Here's how the part is built. I have some questions about the finished solid (model axes, mm). Round coordinates to 2 decimals unless told otherwise and drop trailing zeros. Write each loop counter-clockwise with the first axis right and the second up, starting at its lowest first coordinate (ties: lowest second). Pieces come first, ordered by that corner, then holes. Notation, with made-up numbers: (-22, -40) - (-3, -40) arc R23 cw to (-3, -18) - close; hole circle Ø9 at (25.5, 83.25). An arc over 180 degrees is marked (long way). One line per question, with ' | ' between items. Start each with the question number.
(1) Imagine slicing it at C-C (z = 0.8). Write out the boundary of the cut face in (x, y).
(2) Imagine slicing it at A-A (y = -6.75). Write out the boundary of the cut face in (x, z).
(3) If I drill on L1, parallel to X at y = -5, z = 0.5; L2, parallel to Y at x = 0.1, z = 0.95; L3, parallel to Z at x = -1.6, y = -3, over which ranges is the centre line in solid material (lowest first)?
(4) Imagine slicing it at D-D (x = -0.15). Write out the boundary of the cut face in (y, z).
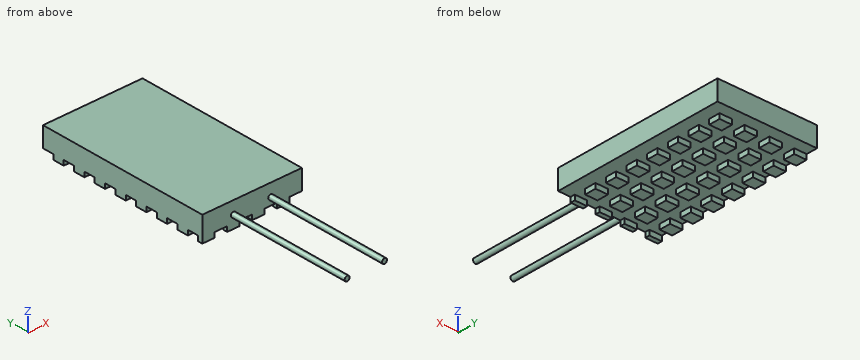
from build123d import *

# Parameters (mm, degrees)
SKETCH_1_W          = 4
SKETCH_1_H          = 7
EXTRUDE_1_DEPTH     = 1
SKETCH_2_W          = 0.5
SKETCH_2_H          = 7
CUT_EXTRUDE_2_DEPTH = 0.2
SKETCH_3_W          = 4
SKETCH_3_H          = 0.454516336
SKETCH_3_H_2        = 0.454516335
CUT_EXTRUDE_4_DEPTH = 0.2
SWEEP_1_PROFILE_R   = 0.1
SWEEP_2_PROFILE_R   = 0.1


with BuildPart() as part:
    # 草图1 → 凸台-拉伸1 (new body)
    with BuildSketch(Plane.XY):
        Rectangle(SKETCH_1_W, SKETCH_1_H)
    extrude(amount=EXTRUDE_1_DEPTH)

    # 草图2 → 切除-拉伸2 (cut)
    with BuildSketch(Plane.XY):
        with Locations((1.75, 0)):
            Rectangle(SKETCH_2_W, SKETCH_2_H)
        with Locations((0.75, 0)):
            Rectangle(SKETCH_2_W, SKETCH_2_H)
        with Locations((-0.25, 0)):
            Rectangle(SKETCH_2_W, SKETCH_2_H)
        with Locations((-1.25, 0)):
            Rectangle(SKETCH_2_W, SKETCH_2_H)
    extrude(amount=CUT_EXTRUDE_2_DEPTH, mode=Mode.SUBTRACT)

    # 草图3 → 切除-拉伸4 (cut)
    with BuildSketch(Plane.XY):
        with Locations((0, 3.272741832)):
            Rectangle(SKETCH_3_W, SKETCH_3_H)
        with Locations((0, 2.363709161)):
            Rectangle(SKETCH_3_W, SKETCH_3_H)
        with Locations((0, 1.45467649)):
            Rectangle(SKETCH_3_W, SKETCH_3_H_2)
        with Locations((0, 0.545643818)):
            Rectangle(SKETCH_3_W, SKETCH_3_H)
        with Locations((0, -0.363388853)):
            Rectangle(SKETCH_3_W, SKETCH_3_H)
        with Locations((0, -1.272421525)):
            Rectangle(SKETCH_3_W, SKETCH_3_H)
        with Locations((0, -2.181454196)):
            Rectangle(SKETCH_3_W, SKETCH_3_H)
        with Locations((0, -3.090486868)):
            Rectangle(SKETCH_3_W, SKETCH_3_H_2)
    extrude(amount=CUT_EXTRUDE_4_DEPTH, mode=Mode.SUBTRACT)

    # 扫描1: sweep along a path in 草图4
    with BuildLine(Plane.XY.offset(0.5)) as sweep_1_path:
        Line((-0.75, -3.5), (-0.75, -8.5))
    # 扫描1 profile (on start of the path) → 扫描1 (sweep)
    with BuildSketch(Plane(origin=(-0.75, -3.5, 0.5), x_dir=(-1, 0, 0), z_dir=(0, -1, 0))):
        Circle(SWEEP_1_PROFILE_R)
    sweep(path=sweep_1_path.line)

    # 扫描2: sweep along a path in 草图11
    with BuildLine(Plane.XY.offset(0.5)) as sweep_2_path:
        Line((0.75, -3.5), (0.75, -8.5))
    # 扫描2 profile (on start of the path) → 扫描2 (sweep)
    with BuildSketch(Plane(origin=(0.75, -3.5, 0.5), x_dir=(-1, 0, 0), z_dir=(0, -1, 0))):
        Circle(SWEEP_2_PROFILE_R)
    sweep(path=sweep_2_path.line)


solid = part.part
Check sheet entries:
1) outline: (-2, -3.5) - (2, -3.5) - (2, 3.5) - (-2, 3.5) - close
2) outline: circle Ø0.2 at (-0.75, 0.5); circle Ø0.2 at (0.75, 0.5)
3) L1: -0.85 to -0.65, 0.65 to 0.85 | L2: -3.5 to 3.5 | L3: 0.2 to 1
4) outline: (-3.5, 0.2) - (3.5, 0.2) - (3.5, 1) - (-3.5, 1) - close
